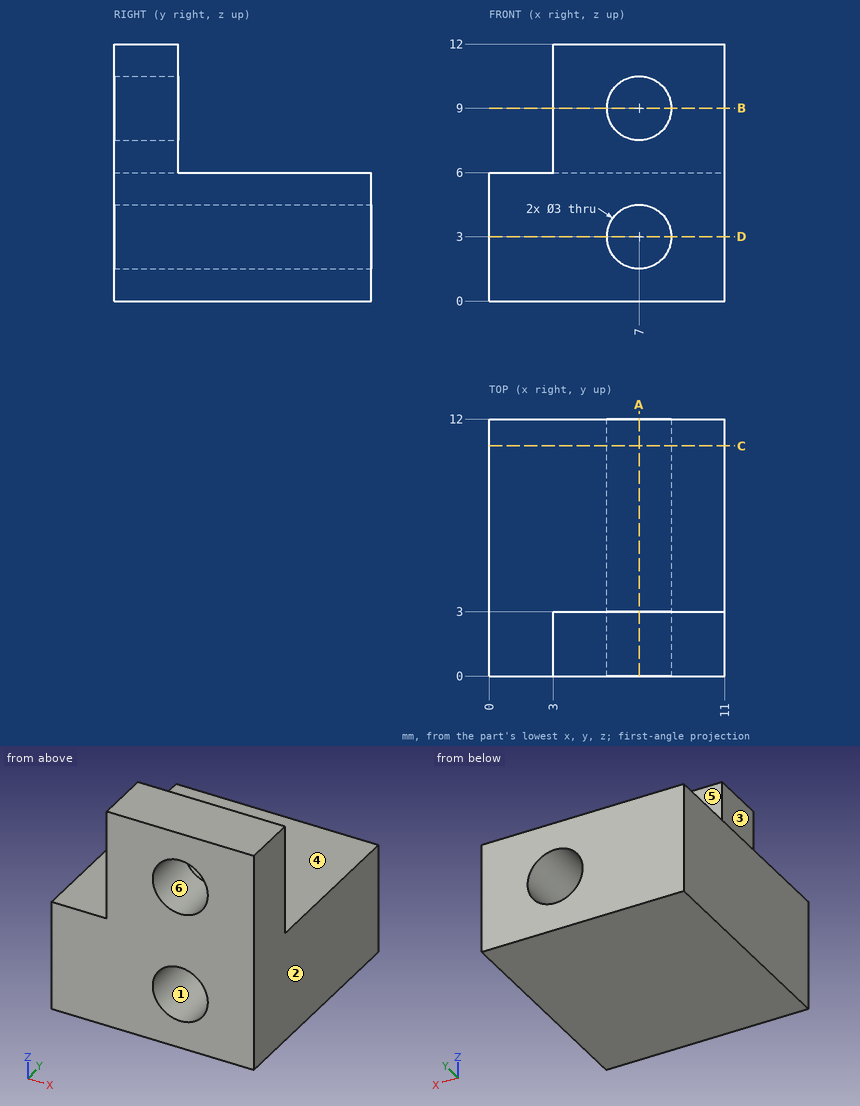
Geometry check sheet. Reference: drawing and pictorial views, mm from the part's lowest x, y, z. A direction names the side the tool comes from. Round coordinates to 2 decimals unless told otherwise and drop trailing zeros. Loops run counter-clockwise (first coordinate to the right, second up) from the corner with the lowest first, then second, coordinate; pieces in that order, holes last. Notation, with made-up numbers: (15.5, 73.5) - (52.5, 73.5) arc R8 cw to (52.5, 78.5) - close; hole circle Ø4 at (25, 16.25). An arc over 180 degrees is marked (long way). Use a Markdown table: item, result.
Q1. Cross-section at B-B on z = 9. Record the cut outline in (x, y).
Solutions:
| item | result |
|---|---|
| outline | (3, 0) - (5.5, 0) - (5.5, 3) - (3, 3) - close; (8.5, 0) - (11, 0) - (11, 3) - (8.5, 3) - close |
Q2. Cross-section at A-A on x = 7. Record the cut outline in (y, z).
Solutions:
| item | result |
|---|---|
| outline | (0, 0) - (12, 0) - (12, 1.5) - (0, 1.5) - close; (0, 4.5) - (12, 4.5) - (12, 6) - (3, 6) - (3, 7.5) - (0, 7.5) - close; (0, 10.5) - (3, 10.5) - (3, 12) - (0, 12) - close |
Q3. Cross-section at C-C on y = 10.75. Record the cut outline in (x, z).
Solutions:
| item | result |
|---|---|
| outline | (0, 0) - (11, 0) - (11, 6) - (0, 6) - close; hole circle Ø3 at (7, 3) |
Q4. Draft check along X on the marked faces 1, 2, 3 and 4. Enter one of: released by +X, released by -X, zero draft, split by the parting line, or undercut.
Solutions:
| item | result |
|---|---|
| face 1 | undercut |
| face 2 | released by +X |
| face 3 | released by -X |
| face 4 | zero draft |
Q5. Go/stop test with flat-tipped pins: P1, Ø0.9, axis at y = 2, z = 7.5, coming from the -X side; P2, Ø2.5, axis at x = 7, z = 3, coming from the -Y side; P3, Ø6.5, axis at x = 8.5, z = 10, coming from the +Y side. Record where each tip stops, or that it passes through.
Solutions:
| item | result |
|---|---|
| P1 | stops at x = 3 |
| P2 | passes through |
| P3 | stops at y = 3 |
Q6. Access from +Z, -Z, +X, -X, +Y, -Y to the whole of each face (thin tool, end or side, straight path). Record for the marked faces 5 and 6.
Solutions:
| item | result |
|---|---|
| face 5 | +Z, +X, -X, +Y |
| face 6 | +Y, -Y |
Q7. Cross-section at D-D on z = 3. Record the cut outline in (x, y), plus the area to 3 significant figures.
Solutions:
| item | result |
|---|---|
| outline | (0, 0) - (5.5, 0) - (5.5, 12) - (0, 12) - close; (8.5, 0) - (11, 0) - (11, 12) - (8.5, 12) - close |
| area | 96.0 mm2 |
Q8. Material ranges on line 1 (Z direction, x = 7, y = 0.6); line 2 (Z direction, x = 7, y = 6.75); line 3 (Z direction, x = 7.5, y = 1.75), recorded low to high.
Solutions:
| item | result |
|---|---|
| line 1 | z = 0 to 1.5, 4.5 to 7.5, 10.5 to 12 |
| line 2 | z = 0 to 1.5, 4.5 to 6 |
| line 3 | z = 0 to 1.59, 4.41 to 7.59, 10.41 to 12 |
